Part print with two shaded views. Sizes in mm from the minimum x, y, z corner. Give positions to 0.01 mm unless a question says otherwise; leave off trailing zeros. Write each loop counter-clockwise with the first axis right and the second up, starting at its lowest first coordinate (ties: lowest second). Pieces come first, ordered by that corner, then holes.
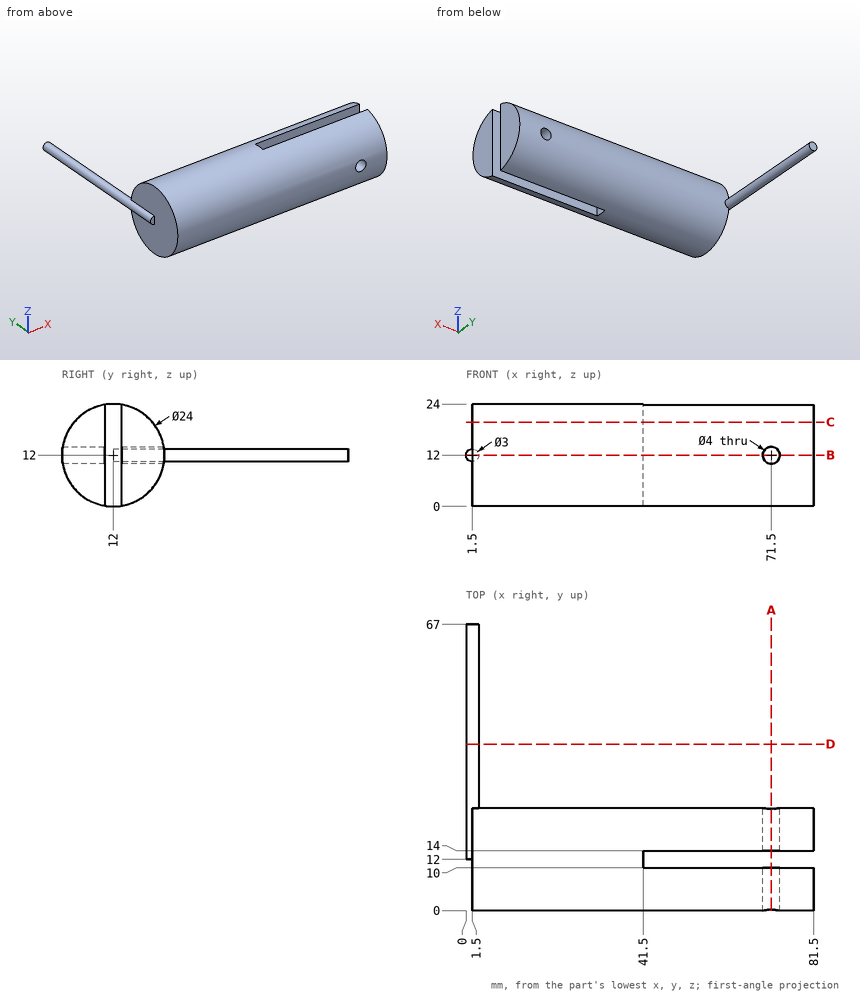
(1) Probe line 1 (X direction, y = 5, z = 12); line 2 (X direction, y = 22, z = 12); line 3 (Y direction, x = 50, z = 11.75). List the from-to ranges inside material, lowest first.
(2) Saw through at D-D, the plane y = 39. List the corners of the cut face in (x, z), plus the area to 3 significant figures.
(3) Drop flat-ended pins along their axis: pin 1 (6.5 mm diameter, centred on x = 71.5, z = 12, fed in from +Y); pin 2 (2 mm diameter, centred on x = 65.5, z = 9.5, fed in from +Y); pin 3 (0.5 mm diameter, centred on x = 0.5, z = 11.5, fed in from -Y). Give the stop position or say it passes through.
(4) Saw through at B-B, the plane z = 12. List the corners of the cut face in (x, y).
(5) Saw through at C-C, the plane z = 19.75. List the corners of the cut face in (x, y).
(6) Saw through at A-A, the plane x = 71.5. List the corners of the cut face in (y, z), plus the area to 3 significant figures.
Computed values:
1. line 1: x = 1.5 to 69.5, 73.5 to 81.5
1. line 2: x = 0 to 69.5, 73.5 to 81.5
1. line 3: y = 0 to 10, 14 to 24
2. outline: circle Ø3 at (1.5, 12)
2. area: 7.07 mm2
3. pin 1: stops at y = 24
3. pin 2: stops at y = 23.91
3. pin 3: stops at y = 12
4. outline: (0, 12) - (1.5, 12) - (1.5, 0) - (69.5, 0) - (69.5, 10) - (41.5, 10) - (41.5, 14) - (69.5, 14) - (69.5, 24) - (3, 24) - (3, 67) - (0, 67) - close; (73.5, 0) - (81.5, 0) - (81.5, 10) - (73.5, 10) - close; (73.5, 14) - (81.5, 14) - (81.5, 24) - (73.5, 24) - close
5. outline: (1.5, 2.84) - (81.5, 2.84) - (81.5, 10) - (41.5, 10) - (41.5, 14) - (81.5, 14) - (81.5, 21.16) - (1.5, 21.16) - close
6. outline: (0.17, 10) arc R12 ccw to (10, 0.17) - (10, 10) - close; (0.17, 14) - (10, 14) - (10, 23.83) arc R12 ccw to start; (14, 0.17) arc R12 ccw to (23.83, 10) - (14, 10) - close; (14, 14) - (23.83, 14) arc R12 ccw to (14, 23.83) - close
6. area: 277 mm2
